Design review of the part built by this model. Coordinates are the model's own, in mm. A direction names the side the tool comes from. Give positions to 0.01 mm unless a question says otherwise; leave off trailing zeros. Loops run counter-clockwise (first coordinate to the right, second up) from the corner with the lowest first, then second, coordinate; pieces in that order, holes last. Notation, with made-up numbers: M 36.5,2 L 43.5,2 A21 cw 43.5,18 Z; hole C 53.5,-29.5 d8. An arc over 180 degrees is marked long. Use one line per item in the form item = value. Start each with the question number.
from build123d import *

# Parameters (mm, degrees)
SKETCH2_W           = 187.00242
SKETCH2_H           = 52.10048
BOSS_EXTRUDE1_DEPTH = 3.175
SKETCH4_R           = 4.074999978
BOSS_EXTRUDE2_DEPTH = 52.10048
FILLET1_R           = 2
FILLET2_R           = 1


with BuildPart() as part:
    # Sketch2 → Boss-Extrude1 (new body)
    with BuildSketch(Plane.XY):
        with Locations((93.50121, 26.05024)):
            Rectangle(SKETCH2_W, SKETCH2_H)
    extrude(amount=BOSS_EXTRUDE1_DEPTH)

    # Sketch4 → Boss-Extrude2 (add, through all)
    # profile 1 of 2: a face of its own
    with BuildSketch(Plane(origin=(0, 52.10048, 0), x_dir=(1, 0, 0), z_dir=(0, 1, 0))):
        with BuildLine():
            Line((53.64742001, 0), (72.70741999, 0))
            Line((72.70741999, 0), (72.70741999, 6.35499999))
            ThreePointArc((72.70741999, 6.35499999), (63.17742, 15.88499998), (53.64742001, 6.35499999))
            Line((53.64742001, 6.35499999), (53.64742001, 0))
        make_face()
        with Locations(Location((63.17742, 6.35499999, 0), (0, 0, 270))):
            Circle(SKETCH4_R, mode=Mode.SUBTRACT)
    # profile 2 of 2: a face of its own
    with BuildSketch(Plane(origin=(0, 52.10048, 0), x_dir=(1, 0, 0), z_dir=(0, 1, 0))):
        with BuildLine():
            Line((132.89542001, 6.35499999), (132.89542001, 0))
            Line((132.89542001, 0), (151.95541999, 0))
            Line((151.95541999, 0), (151.95541999, 6.35499999))
            ThreePointArc((151.95541999, 6.35499999), (142.42542, 15.88499998), (132.89542001, 6.35499999))
        make_face()
        with Locations(Location((142.42542, 6.35499999, 0), (0, 0, 270))):
            Circle(SKETCH4_R, mode=Mode.SUBTRACT)
    extrude(amount=-BOSS_EXTRUDE2_DEPTH)

    # Fillet1
    fillet1_edges = [part.edges().sort_by_distance(p)[0] for p in [
        (72.70741999, 26.05024, 0),
        (53.64742001, 26.05024, 0),
        (151.95541999, 26.05024, 0),
        (132.89542001, 26.05024, 0),
    ]]
    fillet(fillet1_edges, radius=FILLET1_R)

    # Fillet2
    fillet2_edges = [part.edges().sort_by_distance(p)[0] for p in [
        (0, 52.10048, 1.5875),
        (187.00242, 52.10048, 1.5875),
        (187.00242, 0, 1.5875),
        (0, 0, 1.5875),
    ]]
    fillet(fillet2_edges, radius=FILLET2_R)


solid = part.part
Q1. Clearance check with flat-ended pins moving along their axes: pin 1 Ø5 at (y, z) = (33, -4.5) entering from -X; pin 2 Ø4 at (y, z) = (43, -8.5) entering from +X; pin 3 Ø1 at (y, z) = (16.5, -10) entering from -X. State where each tip first meets the part, or that it passes through.
Q2. For faces 5 (the flat face through (25, 26, 0)), 6 (the flat face through (151.955, 26, -4)), 7 (the flat face through (72.707, 26, -4)), 8 (the flat face through (187.002, 26, 2)), list the 3-axis set-ups (+Z, -Z, +X, -X, +Y, -Y) from which the entire face can be reached by the end or side of a thin tool; tool diameter is ignored.
Q3. Wall thickness on probe 1 along X at (y, z) = (12, -4.5); probe 2 along X at (y, z) = (8.5, -7.25); probe 3 along Z at (x, y) = (43, 30.5) (3 decimals): over which ranges is each line inside the solid? List them lowest first.
Q4. Take a section at C-C on y = 6. Give the boundary of the cut face in (x, z) (3 decimals).
Q5. Take a section at A-A on z = -13. Give the boundary of the cut face in (x, y).
Q6. The part is to be moulded in two halves that separate along X. For faces 1 (the cylindrical face through (138.447, 26.415, -7.238)), 2 (the flat face through (92, 26, 3.175)), 3 (the flat face through (102, 26, 0)), 4 (the flat face through (53.647, 26, -4)), say which applies: pulls with the +X half, pulls with the -X half, needs draft (parallel to the pull), parting line crosses it, or undercut.
Q7. Take a section at B-B on x = 61. Give the boundary of the cut face in (y, z) (3 decimals), plus the area to 3 significant figures.
Response values:
q1.pin_1 = 53.65
q1.pin_2 = 151.95
q1.pin_3 = 54.18
q2.face_5 = -Z, -X, +Y, -Y
q2.face_6 = -Z, +X, +Y, -Y
q2.face_7 = -Z, +Y, -Y
q2.face_8 = +Z, -Z, +X, +Y, -Y
q3.probe_1 = 53.65 to 59.55, 66.81 to 72.71, 132.9 to 138.8, 146.05 to 151.96
q3.probe_2 = 53.69 to 59.2, 67.15 to 72.67, 132.94 to 138.45, 146.4 to 151.91
q3.probe_3 = 0 to 3.175
q4.outline = M 0,0 L 51.647,0 A2 cw 53.647,-2 L 53.647,-6.355 A9.53 ccw 72.707,-6.355 L 72.707,-2 A2 cw 74.707,0 L 130.895,0 A2 cw 132.895,-2 L 132.895,-6.355 A9.53 ccw 151.955,-6.355 L 151.955,-2 A2 cw 153.955,0 L 187.002,0 L 187.002,3.175 L 0,3.175 Z; hole C 63.177,-6.355 d8.15; hole C 142.425,-6.355 d8.15
q5.outline = M 56.35,0 L 70.01,0 L 70.01,52.1 L 56.35,52.1 Z; M 135.59,0 L 149.26,0 L 149.26,52.1 L 135.59,52.1 Z
q6.face_1 = undercut
q6.face_2 = needs draft
q6.face_3 = undercut
q6.face_4 = pulls with the -X half
q7.outline = M 0,-15.633 L 52.1,-15.633 L 52.1,-9.799 L 0,-9.799 Z; M 0,-2.911 L 52.1,-2.911 L 52.1,3.175 L 0,3.175 Z
q7.area = 621 mm^2
